```python
from build123d import *

# Parameters (mm, degrees)
F1_DEPTH = 1678
F3_DEPTH = 1678


with BuildPart() as f1:
    # F0 (on Right) → F1 (new body)
    with BuildSketch(Plane.YZ):
        Polygon((0, 25), (0, 0), (0, -25), (597.705221, -25), (820, 618.75), (0, 875), (170, 575), (170, 325), align=None)
    extrude(amount=F1_DEPTH)


with BuildPart() as f3:
    # F2 (on face) → F3 (new body)
    with BuildSketch(Plane.YZ.offset(839)):
        Polygon((170, 575), (0, 875), (-870.606259, 1147.064456), (-870.606259, -25), (0, -25), (0, 0), (0, 25), (170, 325), align=None)
    extrude(amount=-F3_DEPTH)


solid = f3.part
```
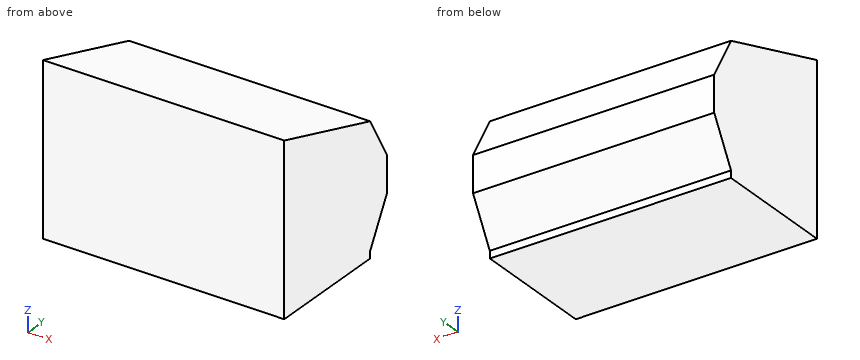
Here's how the part is built. I have some questions about the finished solid (model axes, mm). Give positions to 0.01 mm unless a question says otherwise; leave off trailing zeros. Loops run counter-clockwise (first coordinate to the right, second up) from the corner with the lowest first, then second, coordinate; pieces in that order, holes last. Notation, with made-up numbers: M 20.25,64 L 48.25,64 A16 ccw 48.25,86 Z; hole C 85,20.25 d6. An arc over 180 degrees is marked long. Use one line per item in the form item = value. Start each with the question number.
Q1. If we section it at A-A (x = -505.5): Write out the boundary of the cut face in (y, z), then the cut area to 3 significant figures.
Q2. If we section it at C-C (y = -700): Write out the boundary of the cut face in (x, z).
Q3. Will these pins go through, and if not, where does the flat tip stop? pin 1 Ø6 at (x, y) = (-338.5, -209.5) entering from +Z; pin 2 Ø5 at (x, y) = (-175.5, -113.5) entering from +Z; pin 3 Ø2 at (x, z) = (622.5, 178) entering from +Y.
Q4. If we section it at B-B (z = 920.5): Write out the boundary of the cut face in (x, y), then the cut area to 3 significant figures.
Q5. I need wall thicknesses on line 1 along Z through (x, y) = (-582, -741.5); line 2 along Y through (x, z) = (45.5, 47); line 3 along Y through (x, z) = (258, 60). Which ranges of each line are inside material? Lowest first, please.
Taken from the geometry:
q1.outline = M -870.61,-25 L 0,-25 L 0,25 L 170,325 L 170,575 L 0,875 L -870.61,1147.06 Z
q1.area = 995,000 mm^2
q2.outline = M -839,-25 L 839,-25 L 839,1093.75 L -839,1093.75 Z
q3.pin_1 = 941.41
q3.pin_2 = 911.25
q3.pin_3 = 87.27
q4.outline = M -839,-870.61 L 839,-870.61 L 839,-145.6 L -839,-145.6 Z
q4.area = 1,220,000 mm^2
q5.line_1 = -25 to 1106.72
q5.line_2 = -870.61 to 12.47
q5.line_3 = -870.61 to 19.83
